Source: three-view drawing plus pictorial views. Frame: mm from the lowest corner of the part. A direction names the side the tool comes from. Give positions to 0.01 mm unless a question says otherwise; leave off trailing zeros. Order: outer loops, then holes, each group sorted by start corner. A loop starts at its lowest first (then second) coordinate and runs counter-clockwise, first axis right, second up.
1) Section D-D, the plane z = 6. Return loops of the section in (x, y), plus the area to 3 significant figures.
2) First-contact query: P1, Ø8, axis at x = 73.5, y = 70.5, coming from the -Z side. Flat tip, straight axial feed; report the tip coordinate or a pass-through.
3) Section A-A, the plane x = 98. Return loops of the section in (y, z), plus the area to 3 significant figures.
4) Section C-C, the plane y = 10. Return loops of the section in (x, z), plus the area to 3 significant figures.
5) Section B-B, the plane z = 11.75. Return loops of the section in (x, y).
6) Material intervals for line 1 (X direction, y = 47, z = 5.5); line 2 (X direction, y = 31, z = 1.75); line 3 (Z direction, x = 102, y = 9), sorted ascending.
7) Draft query along X for the marked faces 3, 4 and 5. Return one class per face: released by +X, released by -X, zero draft, split by the parting line, or undercut.
8) Access query for the marked faces 1 and 2. Directions: +Z, -Z, +X, -X, +Y, -Y. A direction counts if a zero-diameter tool reaches every point of the face in a straight line with its end or side. Return the directions, or none.
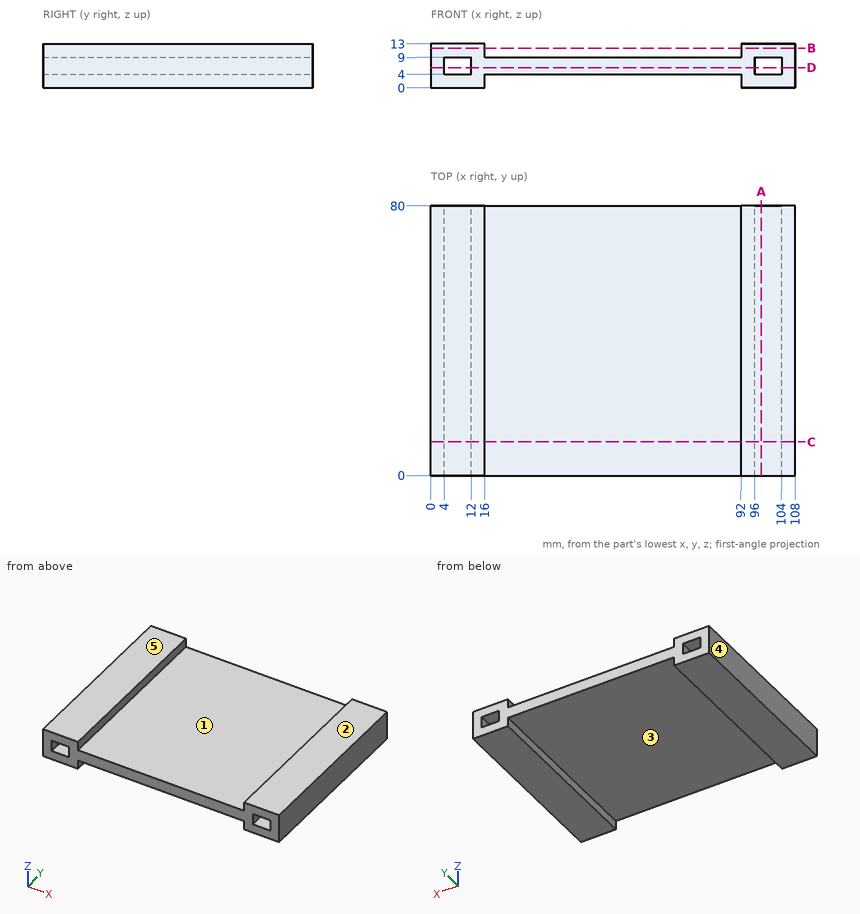
From the geometry:
1. outline: (0, 0) - (4, 0) - (4, 80) - (0, 80) - close; (12, 0) - (96, 0) - (96, 80) - (12, 80) - close; (104, 0) - (108, 0) - (108, 80) - (104, 80) - close
1. area: 7,360 mm2
2. P1: stops at z = 4
3. outline: (0, 0) - (80, 0) - (80, 4) - (0, 4) - close; (0, 9) - (80, 9) - (80, 13) - (0, 13) - close
3. area: 640 mm2
4. outline: (0, 0) - (16, 0) - (16, 4) - (92, 4) - (92, 0) - (108, 0) - (108, 13) - (92, 13) - (92, 9) - (16, 9) - (16, 13) - (0, 13) - close; hole (4, 4) - (12, 4) - (12, 9) - (4, 9) - close; hole (96, 4) - (104, 4) - (104, 9) - (96, 9) - close
4. area: 716 mm2
5. outline: (0, 0) - (16, 0) - (16, 80) - (0, 80) - close; (92, 0) - (108, 0) - (108, 80) - (92, 80) - close
6. line 1: x = 0 to 4, 12 to 96, 104 to 108
6. line 2: x = 0 to 16, 92 to 108
6. line 3: z = 0 to 4, 9 to 13
7. face 3: undercut
7. face 4: released by -X
7. face 5: zero draft
8. face 1: +Z, +Y, -Y
8. face 2: +Z, +X, -X, +Y, -Y
